Check sheet for the modelled part. Datum: model origin and axes. Units: mm. Give positions to 0.01 mm unless a question says otherwise; leave off trailing zeros. Order: outer loops, then holes, each group sorted by start corner. A loop starts at its lowest first (then second) coordinate and runs counter-clockwise, first axis right, second up.
```python
from build123d import *

# Parameters (mm, degrees)
SKETCH1_W                   = 22.8092
SKETCH1_H                   = 22.8092
SKETCH1_W_2                 = 20.1422
SKETCH1_H_2                 = 20.1422
BOSS_EXTRUDE1_DEPTH         = 1303.02
FILLET1_R                   = 2.54
F_1_4_0_25_DIAMETER_HOLE1_D = 6.35
F_1_4_CLEARANCE_HOLE1_D     = 6.7564


with BuildPart() as part:
    # Sketch1 → Boss-Extrude1 (new body)
    with BuildSketch(Plane(origin=(0, 0, 0), x_dir=(1, 0, 0), z_dir=(0, 1, 0))):
        Rectangle(SKETCH1_W, SKETCH1_H)
        Rectangle(SKETCH1_W_2, SKETCH1_H_2, mode=Mode.SUBTRACT)
    extrude(amount=BOSS_EXTRUDE1_DEPTH)

    # Fillet1
    fillet1_edges = [part.edges().sort_by_distance(p)[0] for p in [
        (11.4046, 651.51, 11.4046),
        (-11.4046, 651.51, 11.4046),
        (-11.4046, 651.51, -11.4046),
        (11.4046, 651.51, -11.4046),
    ]]
    fillet(fillet1_edges, radius=FILLET1_R)

    # 1/4 (0.25) Diameter Hole1 (through all)
    with Locations(Plane(origin=(0, 0, 0), x_dir=(-1, 0, 0), z_dir=(0, -1, 0))):
        with Locations((0, 0)):
            Hole(F_1_4_0_25_DIAMETER_HOLE1_D / 2)

    # 1/4 Clearance Hole1 (through all)
    with Locations(Plane(origin=(11.4046, 0, 0), x_dir=(0, 0, -1), z_dir=(1, 0, 0))):
        with Locations((0, 1287.145)):
            Hole(F_1_4_CLEARANCE_HOLE1_D / 2)


solid = part.part
```
Q1. Material ranges on line 1 (Z direction, x = -4.5, y = 1076); line 2 (Y direction, x = -10.45, z = 0); line 3 (X direction, y = 566, z = -9.5), recorded low to high.
Q2. Sectioned sample at A-A, the plane x = 4.25. Record the cut outline in (y, z).
Q3. Draft check along X on faces 1 (the flat face through (10.071, 642, 0)), 2 (the flat face through (-10.071, 642, 0)). Enter one of: pulls with the +X half, pulls with the -X half, needs draft (parallel to the pull), parting line crosses it, or undercut.
Q4. Go/stop test with a flat-tipped pin: P1, Ø9, axis at y = 1287.145, z = 0, coming from the +X side. Record where the tip stops, or that it passes through.
Q5. Sectioned sample at B-B, the plane y = 649. Record the cut outline in (x, z), plus the area to 3 significant figures.
Filled in:
1. line 1: z = -11.4 to -10.07, 10.07 to 11.4
1. line 2: y = 0 to 1283.77, 1290.52 to 1303.02
1. line 3: x = -11.32 to -10.07, 10.07 to 11.32
2. outline: (0, -11.4) - (1303.02, -11.4) - (1303.02, -10.07) - (0, -10.07) - close; (0, 10.07) - (1303.02, 10.07) - (1303.02, 11.4) - (0, 11.4) - close
3. face 1: undercut
3. face 2: undercut
4. P1: stops at x = 11.4
5. outline: (-11.4, -8.86) arc R2.54 ccw to (-8.86, -11.4) - (8.86, -11.4) arc R2.54 ccw to (11.4, -8.86) - (11.4, 8.86) arc R2.54 ccw to (8.86, 11.4) - (-8.86, 11.4) arc R2.54 ccw to (-11.4, 8.86) - close; hole (-10.07, -10.07) - (10.07, -10.07) - (10.07, 10.07) - (-10.07, 10.07) - close
5. area: 109 mm2
